Here's how the part is built. I have some questions about the finished solid (model axes, mm). A direction names the side the tool comes from. Give positions to 0.01 mm unless a question says otherwise; leave off trailing zeros. Write each loop counter-clockwise with the first axis right and the second up, starting at its lowest first coordinate (ties: lowest second). Pieces come first, ordered by that corner, then holes. Notation, with made-up numbers: (37.5, -20) -> (66.5, -20) arc R27 cw to (66.5, -4) -> close; hole circle Ø11 at (62, 19.25). An arc over 180 degrees is marked (long way). Return JSON: item names as keys, results as strings.
from build123d import *

# Parameters (mm, degrees)
EXTRUDE_DEPTH = 0.7


with BuildPart() as part:
    # Sketch → Extrude (new body)
    with BuildSketch(Plane.XY):
        with BuildLine():
            ThreePointArc((5.5, -8.050621), (0, 9.75), (-5.5, -8.050621))
            Line((-5.5, -8.050621), (-4.25, -4.62132))
            Line((-4.25, -2.12132), (-4.25, -4.62132))
            ThreePointArc((4.25, -2.12132), (0, 4.75), (-4.25, -2.12132))
            Line((4.25, -2.12132), (4.25, -4.62132))
            Line((4.25, -4.62132), (5.5, -8.050621))
        make_face()
    extrude(amount=EXTRUDE_DEPTH)


solid = part.part
1. Suppose I cut it at D-D, the plane x = 0. List the corners of the cut face in (y, z) for me, and give its area (3 significant figures).
Taken from the geometry:
{"outline": "(4.75, 0) -> (9.75, 0) -> (9.75, 0.7) -> (4.75, 0.7) -> close", "area": "3.50 mm²"}
2. Which directions (+Z, -Z, +X, -X, +Y, -Y) give clear straight access to the entire face, cutting with the end or side of a thin tool? Please do faces 1 (the face through (0, 5, 0.7)), 2 (the face through (-4.9, -6.4, 0.3)).
Taken from the geometry:
{"face 1": "+Z, +X, -X, +Y, -Y", "face 2": "+Z, -Z, -Y"}
3. Suppose I cut it at C-C, the plane z = 0.15. List the corners of the cut face in (x, y) for me.
Taken from the geometry:
{"outline": "(-5.5, -8.05) -> (-4.25, -4.62) -> (-4.25, -2.12) arc R4.75 cw (long way) to (4.25, -2.12) -> (4.25, -4.62) -> (5.5, -8.05) arc R9.75 ccw (long way) to start"}
4. Suppose I cut it at A-A, the plane y = 0. List the corners of the cut face in (x, z) for me.
Taken from the geometry:
{"outline": "(-9.75, 0) -> (-4.75, 0) -> (-4.75, 0.7) -> (-9.75, 0.7) -> close; (4.75, 0) -> (9.75, 0) -> (9.75, 0.7) -> (4.75, 0.7) -> close"}
5. If we mould it in two halves opening along Y, with no side actions, what happens to faces 3 (the face through (0.135, 4.748, 0.345)), 4 (the face through (4.866, -6.312, 0.345)), 5 (the face through (0.347, 9.744, 0.345))? For each: released by +Y, released by -Y, zero draft, split by the parting line, or undercut.
Taken from the geometry:
{"face 3": "undercut", "face 4": "released by -Y", "face 5": "split by the parting line"}
6. Suppose I cut it at B-B, the plane x = -4.5. List the corners of the cut face in (y, z) for me, and give its area (3 significant figures).
Taken from the geometry:
{"outline": "(-5.31, 0) -> (-1.52, 0) -> (-1.52, 0.7) -> (-5.31, 0.7) -> close; (1.52, 0) -> (8.65, 0) -> (8.65, 0.7) -> (1.52, 0.7) -> close", "area": "7.64 mm²"}
7. If I drill on line 1 (X direction, y = -5.75, z = 0.1); line 2 (X direction, y = -4, z = 0.2); line 3 (Y direction, x = -3.5, z = 0.45), over which ranges is the centre line in solid material (lowest first)? Write a range as [from, to].
Taken from the geometry:
{"line 1": "x = [-7.87, -4.66], [4.66, 7.87]", "line 2": "x = [-8.89, -4.25], [4.25, 8.89]", "line 3": "y = [3.21, 9.1]"}
